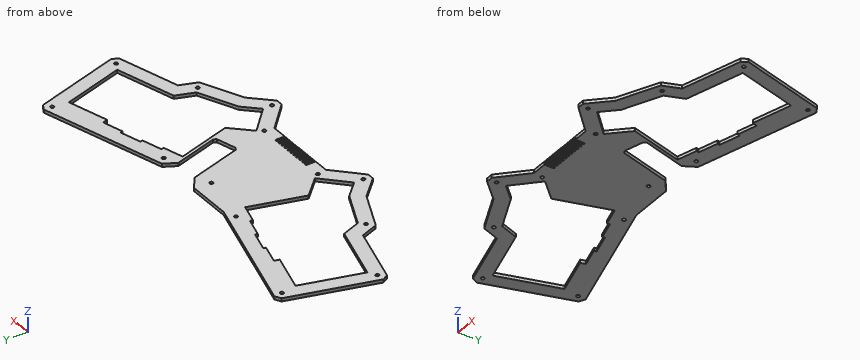
```python
from build123d import *

# Parameters (mm, degrees)
ESQUISSE1_R             = 1.6
BOSS_EXTRU_1_DEPTH      = 3
ENL_V_MAT_EXTRU_1_DEPTH = 10


with BuildPart() as part:
    # Esquisse1 → Boss.-Extru.1 (new body)
    with BuildSketch(Plane.XY):
        Polygon((-119.070790786, -62.796362516), (-130.649820486, -22.415487094), (-124.479201425, -11.283395628), (-113.904378452, -8.251113935), (-107.178924408, -6.322621021), (-11.444293109, 21.123080509), (-5.984240232, 18.096325283), (16.733855492, -61.131089881), (13.707363231, -66.591026451), (-42.255771499, -82.638197107), (-48.091810819, -98.561018129), (-85.310364869, -115.48724507), (-102.69792658, -133.444615579), (-108.937044092, -133.542771169), (-132.888887149, -110.350948678), (-202.701632594, -110.350948678), (-226.653475651, -133.542771169), (-232.892593163, -133.444615579), (-250.280154874, -115.48724507), (-287.498708924, -98.561018129), (-293.334748244, -82.638197107), (-349.297882974, -66.591026451), (-352.324375235, -61.131089881), (-329.606279511, 18.096325283), (-324.146226634, 21.123080509), (-228.411595335, -6.322621021), (-221.686141291, -8.251113935), (-206.165691337, -12.701531345), (-165.848732708, -12.701531345), (-154.419403971, -21.314148304), (-140.742647218, -69.010667349), (-138.268849115, -70.381916029), (-120.442039466, -65.27016062), align=None)
        with Locations((-12.000450916, 13.68165837)):
            Circle(ESQUISSE1_R, mode=Mode.SUBTRACT)
        with Locations((-118.757933777, -16.924131519)):
            Circle(ESQUISSE1_R, mode=Mode.SUBTRACT)
        with Locations((9.292284284, -60.574933915)):
            Circle(ESQUISSE1_R, mode=Mode.SUBTRACT)
        with Locations((-53.656180266, -93.401689518)):
            Circle(ESQUISSE1_R, mode=Mode.SUBTRACT)
        with Locations((-105.923928137, -126.713325795)):
            Circle(ESQUISSE1_R, mode=Mode.SUBTRACT)
        with Locations((-131.530967037, -101.880200807)):
            Circle(ESQUISSE1_R, mode=Mode.SUBTRACT)
        with Locations((-204.059552706, -101.880200807)):
            Circle(ESQUISSE1_R, mode=Mode.SUBTRACT)
        with Locations((-229.666591606, -126.713325795)):
            Circle(ESQUISSE1_R, mode=Mode.SUBTRACT)
        with Locations((-281.934339477, -93.401689518)):
            Circle(ESQUISSE1_R, mode=Mode.SUBTRACT)
        with Locations((-344.882804027, -60.574933915)):
            Circle(ESQUISSE1_R, mode=Mode.SUBTRACT)
        with Locations((-216.832585966, -16.924131519)):
            Circle(ESQUISSE1_R, mode=Mode.SUBTRACT)
        with Locations((-323.590068827, 13.68165837)):
            Circle(ESQUISSE1_R, mode=Mode.SUBTRACT)
        with Locations((-167.795259872, -27.605548894)):
            Circle(ESQUISSE1_R, mode=Mode.SUBTRACT)
        Polygon((-128.0696158, -96.878899722), (-106.057456456, -118.225792128), (-92.935433745, -104.673746846), (-58.425639792, -88.979407851), (-52.188593581, -71.96249534), (1.870889973, -56.461187875), (-14.186085737, -0.463858857), (-50.716621092, -10.938821309), (-52.025991399, -6.372504389), (-70.291259076, -11.609985616), (-70.910965859, -9.448811229), (-90.137733677, -14.960840928), (-89.517720268, -17.123084647), (-107.782987945, -22.360565873), (-107.093845678, -24.763890567), (-125.358331696, -30.001147656), (-111.200088958, -79.377961929), (-127.377713529, -96.161100182), align=None, mode=Mode.SUBTRACT)
        Polygon((-224.390430785, -79.377961929), (-208.212806214, -96.161100182), (-207.491865187, -96.85509979), (-208.236606037, -97.572971364), (-229.533063287, -118.225792128), (-242.655085998, -104.673746846), (-277.164879951, -88.979407851), (-283.401926162, -71.96249534), (-337.461409717, -56.461187875), (-321.404434006, -0.463858857), (-284.873898651, -10.938821309), (-283.564528345, -6.372504389), (-265.299260667, -11.609985616), (-264.679553884, -9.448811229), (-245.452786066, -14.960840928), (-246.072799476, -17.123084647), (-227.807531798, -22.360565873), (-228.496674065, -24.763890567), (-210.232188047, -30.001147656), align=None, mode=Mode.SUBTRACT)
    extrude(amount=BOSS_EXTRU_1_DEPTH)

    # Esquisse2 → Enlèv. mat.-Extru.1 (cut)
    with BuildSketch(Plane.XY.offset(3)):
        with BuildLine():
            Line((-168.795259872, -110.350948678), (-168.795259872, -102.350948678))
            ThreePointArc((-168.795259872, -102.350948678), (-167.795259872, -101.350948678), (-166.795259872, -102.350948678))
            Line((-166.795259872, -102.350948678), (-166.795259872, -110.350948678))
            ThreePointArc((-166.795259872, -110.350948678), (-167.795259872, -111.350948678), (-168.795259872, -110.350948678))
        make_face()
        with BuildLine():
            Line((-164.795259872, -110.350948678), (-164.795259872, -102.350948678))
            ThreePointArc((-164.795259872, -102.350948678), (-163.795259872, -101.350948678), (-162.795259872, -102.350948678))
            Line((-162.795259872, -102.350948678), (-162.795259872, -110.350948678))
            ThreePointArc((-162.795259872, -110.350948678), (-163.795259872, -111.350948678), (-164.795259872, -110.350948678))
        make_face()
        with BuildLine():
            Line((-160.795259872, -110.350948678), (-160.795259872, -102.350948678))
            ThreePointArc((-160.795259872, -102.350948678), (-159.795259872, -101.350948678), (-158.795259872, -102.350948678))
            Line((-158.795259872, -102.350948678), (-158.795259872, -110.350948678))
            ThreePointArc((-158.795259872, -110.350948678), (-159.795259872, -111.350948678), (-160.795259872, -110.350948678))
        make_face()
        with BuildLine():
            Line((-156.795259872, -110.350948678), (-156.795259872, -102.350948678))
            ThreePointArc((-156.795259872, -102.350948678), (-155.795259872, -101.350948678), (-154.795259872, -102.350948678))
            Line((-154.795259872, -102.350948678), (-154.795259872, -110.350948678))
            ThreePointArc((-154.795259872, -110.350948678), (-155.795259872, -111.350948678), (-156.795259872, -110.350948678))
        make_face()
        with BuildLine():
            Line((-152.795259872, -110.350948678), (-152.795259872, -102.350948678))
            ThreePointArc((-152.795259872, -102.350948678), (-151.795259872, -101.350948678), (-150.795259872, -102.350948678))
            Line((-150.795259872, -102.350948678), (-150.795259872, -110.350948678))
            ThreePointArc((-150.795259872, -110.350948678), (-151.795259872, -111.350948678), (-152.795259872, -110.350948678))
        make_face()
        with BuildLine():
            Line((-148.795259872, -110.350948678), (-148.795259872, -102.350948678))
            ThreePointArc((-148.795259872, -102.350948678), (-147.795259872, -101.350948678), (-146.795259872, -102.350948678))
            Line((-146.795259872, -102.350948678), (-146.795259872, -110.350948678))
            ThreePointArc((-146.795259872, -110.350948678), (-147.795259872, -111.350948678), (-148.795259872, -110.350948678))
        make_face()
        with BuildLine():
            Line((-172.795259872, -110.350948678), (-172.795259872, -102.350948678))
            ThreePointArc((-172.795259872, -102.350948678), (-171.795259872, -101.350948678), (-170.795259872, -102.350948678))
            Line((-170.795259872, -102.350948678), (-170.795259872, -110.350948678))
            ThreePointArc((-170.795259872, -110.350948678), (-171.795259872, -111.350948678), (-172.795259872, -110.350948678))
        make_face()
        with BuildLine():
            Line((-176.795259872, -110.350948678), (-176.795259872, -102.350948678))
            ThreePointArc((-176.795259872, -102.350948678), (-175.795259872, -101.350948678), (-174.795259872, -102.350948678))
            Line((-174.795259872, -102.350948678), (-174.795259872, -110.350948678))
            ThreePointArc((-174.795259872, -110.350948678), (-175.795259872, -111.350948678), (-176.795259872, -110.350948678))
        make_face()
        with BuildLine():
            Line((-180.795259872, -110.350948678), (-180.795259872, -102.350948678))
            ThreePointArc((-180.795259872, -102.350948678), (-179.795259872, -101.350948678), (-178.795259872, -102.350948678))
            Line((-178.795259872, -102.350948678), (-178.795259872, -110.350948678))
            ThreePointArc((-178.795259872, -110.350948678), (-179.795259872, -111.350948678), (-180.795259872, -110.350948678))
        make_face()
        with BuildLine():
            Line((-184.795259872, -110.350948678), (-184.795259872, -102.350948678))
            ThreePointArc((-184.795259872, -102.350948678), (-183.795259872, -101.350948678), (-182.795259872, -102.350948678))
            Line((-182.795259872, -102.350948678), (-182.795259872, -110.350948678))
            ThreePointArc((-182.795259872, -110.350948678), (-183.795259872, -111.350948678), (-184.795259872, -110.350948678))
        make_face()
        with BuildLine():
            Line((-188.795259872, -110.350948678), (-188.795259872, -102.350948678))
            ThreePointArc((-188.795259872, -102.350948678), (-187.795259872, -101.350948678), (-186.795259872, -102.350948678))
            Line((-186.795259872, -102.350948678), (-186.795259872, -110.350948678))
            ThreePointArc((-186.795259872, -110.350948678), (-187.795259872, -111.350948678), (-188.795259872, -110.350948678))
        make_face()
    extrude(amount=-ENL_V_MAT_EXTRU_1_DEPTH, mode=Mode.SUBTRACT)


solid = part.part
```
Here's how the part is built. I have some questions about the finished solid (model axes, mm). Round coordinates to 2 decimals unless told otherwise and drop trailing zeros. Loops run counter-clockwise (first coordinate to the right, second up) from the corner with the lowest first, then second, coordinate; pieces in that order, holes last.
1. Suppose I cut it at C-C, the plane z = 0.8. Give the number of separate pieces and of enclosed holes in the cut face, and give its area (3 significant figures).
Answers:
separate pieces: 1
enclosed holes: 15
area: 17,900 mm2
2. Suppose I cut it at B-B, the plane x = -75. Please give me the cut outline in (y, z).
Answers:
outline: (-110.8, 0) - (-96.52, 0) - (-96.52, 3) - (-110.8, 3) - close; (-10.62, 0) - (2.9, 0) - (2.9, 3) - (-10.62, 3) - close
3. Suppose I cut it at A-A, the plane y = 3.5. Please give me the cut outline in (x, z).
Answers:
outline: (-333.79, 0) - (-262.67, 0) - (-262.67, 3) - (-333.79, 3) - close; (-72.92, 0) - (-1.8, 0) - (-1.8, 3) - (-72.92, 3) - close
4. If I drill on probe 1 along X at (y, z) = (-35, 2.5); probe 2 along X at (y, z) = (-89, 0.4); probe 3 along X at (y, z) = (-36, 1.2), over which ranges is the centre line in solid material (lowest first)?
Answers:
probe 1: x = -344.83 to -331.31, -211.67 to -150.5, -127.04 to -123.92, -4.28 to 9.24
probe 2: x = -291 to -277.12, -215.12 to -120.47, -58.47 to -44.59
probe 3: x = -345.12 to -331.59, -211.95 to -150.21, -126.75 to -123.64, -4 to 9.53
5. Will these pins go through, and if not, where does the flat tip stop? pin 1 (0.9 mm diameter, centred on y = -108, z = 2, fed in from -X); pin 2 (0.9 mm diameter, centred on x = -190.5, z = 1, fed in from +Y); pin 3 (0.9 mm diameter, centred on y = -107, z = 1.5, fed in from -X).
Answers:
pin 1: stops at x = -267.73
pin 2: stops at y = -12.7
pin 3: stops at x = -269.93
